The listing builds one solid part. Answer for the finished solid, in the listing's coordinates (mm). Face numbers are marked on the shaded views. A direction names the side the tool comes from. Coordinates: 2 decimals unless noted, no trailing zeros. Order: outer loops, then holes, each group sorted by start corner. A loop starts at its lowest first (then second) coordinate and runs counter-clockwise, first axis right, second up. Notation, with made-up numbers: (31, 49.5) -> (79, 49.5) arc R32 cw to (79, 82.5) -> close; hole circle Ø1 at (-12, -31.5). An arc over 180 degrees is marked (long way). Answer in a Markdown table with one row per item.
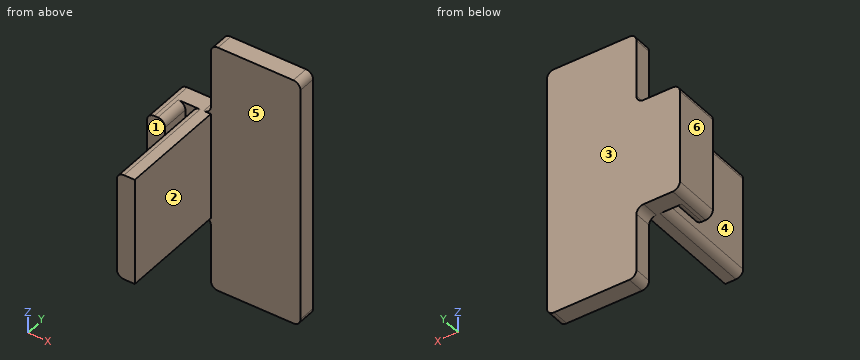
```python
from build123d import *

# Parameters (mm, degrees)
F1_DEPTH = 15
F0_W     = 25
F0_H     = 5
F2_DEPTH = 35
F3_R     = 2


with BuildPart() as f1:
    # F0 (on Top) → F1 (new body, symmetric)
    with BuildSketch(Plane.XY):
        Polygon((-12.1, 0), (-12.1, -13), (-7.1, -13), (-7.1, -5), (-5, -5), (-5, -35), (0, -35), (0, -5), (0, 0), align=None)
    extrude(amount=F1_DEPTH, both=True)

    # F0 (on Top) → F2 (join, symmetric)
    with BuildSketch(Plane.XY):
        with Locations((12.5, -2.5)):
            Rectangle(F0_W, F0_H)
    extrude(amount=F2_DEPTH, both=True)

    # F3
    f3_edges = [f1.edges().sort_by_distance(p)[0] for p in [
        (0, -2.5, 15),
        (0, -2.5, -15),
        (0, -2.5, -35),
        (0, -2.5, 35),
        (25, -2.5, 35),
        (25, -2.5, -35),
        (-12.1, -6.5, 15),
        (-5, -20, 15),
        (-7.1, -9, 15),
        (-5, -20, -15),
        (-12.1, -6.5, -15),
        (-7.1, -9, -15),
    ]]
    fillet(f3_edges, radius=F3_R)


solid = f1.part
```
(1) Find the intervals of material crossed by line 1 along Y through (x, z) = (7, 26); line 2 along Z through (x, y) = (-3, -7), in increasing order. Write a range as from..to.
Check values:
| item | result |
|---|---|
| line 1 | -5..0 |
| line 2 | -15..15 |
(2) Flat-ended cylindrical pins translate along their axes: pin 1 (8 mm diameter, centred on x = 19, z = 6, fed in from +Y); pin 2 (10 mm diameter, centred on x = -8.5, y = -27.5, fed in from -Z); pin 3 (11 mm diameter, centred on x = -6.5, y = -24.5, fed in from +Z); pin 4 (10 mm diameter, centred on y = -24, z = 19.5, fed in from +X). Find the tip coordinate at first contact, or state that the pin passes through.
Check values:
| item | result |
|---|---|
| pin 1 | y = 0 |
| pin 2 | z = -14.94 |
| pin 3 | z = 15 |
| pin 4 | x = 0 |
(3) For a pull along X with two mould halves and no side action, classify the marked faces 4, 5 and 6 as released by +X, released by -X, zero draft, split by the parting line, or undercut.
Check values:
| item | result |
|---|---|
| face 4 | undercut |
| face 5 | zero draft |
| face 6 | released by -X |
(4) A cutting plane is placed at B-B, the plane y = -24. Determine the outline of the cut face in (x, z).
Check values:
| item | result |
|---|---|
| outline | (-5, -13) arc R2 ccw to (-3, -15) -> (0, -15) -> (0, 15) -> (-3, 15) arc R2 ccw to (-5, 13) -> close |
(5) A cutting plane is placed at D-D, the plane x = 22. Determine the outline of the cut face in (y, z).
Check values:
| item | result |
|---|---|
| outline | (-5, -35) -> (0, -35) -> (0, 35) -> (-5, 35) -> close |
(6) Which of the six approach directions +Z, -Z, +X, -X, +Y, -Y give full straight-line access (tool end or side, diameter ignored) to the marked faces 1, 2 and 3?
Check values:
| item | result |
|---|---|
| face 1 | +Z, -Z, -X, -Y |
| face 2 | +Z, -Z, +X, -Y |
| face 3 | +Z, -Z, +X, -X, +Y |
(7) A cutting plane is placed at A-A, the plane y = -7. Determine the outline of the cut face in (x, z).
Check values:
| item | result |
|---|---|
| outline | (-12.1, -13) arc R2 ccw to (-10.1, -15) -> (-9.1, -15) arc R2 ccw to (-7.1, -13) -> (-7.1, 13) arc R2 ccw to (-9.1, 15) -> (-10.1, 15) arc R2 ccw to (-12.1, 13) -> close; (-5, -13) arc R2 ccw to (-3, -15) -> (0, -15) -> (0, 15) -> (-3, 15) arc R2 ccw to (-5, 13) -> close |
(8) A cutting plane is placed at C-C, the plane z = -1. Determine the outline of the cut face in (x, y).
Check values:
| item | result |
|---|---|
| outline | (-12.1, -13) -> (-7.1, -13) -> (-7.1, -5) -> (-5, -5) -> (-5, -35) -> (0, -35) -> (0, -5) -> (25, -5) -> (25, 0) -> (-12.1, 0) -> close |
